```python
from build123d import *

# Parameters (mm, degrees)
SKETCH1_R            = 17.5
SKETCH1_R_2          = 15
BOSS_EXTRUDE1_DEPTH  = 80
CUT_SWEEP3_PROFILE_R = 2
FILLET2_R            = 2


with BuildPart() as part:
    # Sketch1 → Boss-Extrude1 (new body)
    with BuildSketch(Plane.XY):
        with BuildLine():
            Line((-17.5, 72.107864376), (-17.5, 63.75))
            Line((-17.5, 63.75), (-17.5, -66.25))
            Line((-17.5, -66.25), (-17.5, -76.567541634))
            ThreePointArc((-17.5, -76.567541634), (0, -106.25), (17.5, -76.567541634))
            Line((17.5, -76.567541634), (77.5, -76.567541634))
            Line((77.5, -76.567541634), (77.5, 72.107864376))
            Line((77.5, 72.107864376), (17.5, 72.107864376))
            ThreePointArc((17.5, 72.107864376), (0, 108.75), (-17.5, 72.107864376))
        make_face()
        with Locations((0, 86.25)):
            Circle(SKETCH1_R, mode=Mode.SUBTRACT)
        with Locations((0, -86.25)):
            Circle(SKETCH1_R_2, mode=Mode.SUBTRACT)
    extrude(amount=BOSS_EXTRUDE1_DEPTH)

    # Sketch9 → Cut-Revolve1 (revolve, cut)
    with BuildSketch(Plane.XY.offset(40), mode=Mode.PRIVATE) as cut_revolve1_sk:
        Polygon((-7.353554792, 47.770161371), (-7.353554792, 17.770161371), (6.646445208, 17.770161371), (6.646445208, 45.270161371), (12.283096941, 45.270161371), (12.283096941, 30.270161371), (62.283096941, 30.270161371), (62.283096941, 47.770161371), align=None)
    revolve(cut_revolve1_sk.sketch.rotate(Axis((-48.211470633, 47.770161371, 40), (1, 0, 0)), 270), axis=Axis((-48.211470633, 47.770161371, 40), (1, 0, 0)), mode=Mode.SUBTRACT)

    # Sketch38 → Cut-Revolve3 (revolve, cut)
    with BuildSketch(Plane.XY.offset(40), mode=Mode.PRIVATE) as cut_revolve3_sk:
        Polygon((17, 0), (17, 12.5), (22.475179435, 12.5), (22.475179435, 17.5), (102.052596933, 17.5), (102.052596933, 0), align=None)
    revolve(cut_revolve3_sk.sketch.rotate(Axis((102.052596933, 0, 40), (-1, 0, 0)), 90), axis=Axis((102.052596933, 0, 40), (-1, 0, 0)), mode=Mode.SUBTRACT)

    # Cut-Sweep3: sweep along a path in Sketch60
    with BuildLine(Plane.XY.offset(40)) as cut_sweep3_path:
        Line((57.751179251, 47.84482156), (68.211067836, 47.84482156))
        Line((68.211067836, 47.84482156), (68.211067836, 23.494918311))
        Line((68.211067836, 23.494918311), (19.159559926, 23.494918311))
        Line((19.159559926, 23.494918311), (19.159559926, 12.07117719))
    # Cut-Sweep3 profile (on start of the path) → Cut-Sweep3 (sweep, cut)
    with BuildSketch(Plane(origin=(57.751179251, 47.84482156, 40), x_dir=(0, 0, 1), z_dir=(1, 0, 0))):
        Circle(CUT_SWEEP3_PROFILE_R)
    sweep(path=cut_sweep3_path.line, transition=Transition.RIGHT, mode=Mode.SUBTRACT)

    # Fillet2
    fillet2_edges = [part.edges().sort_by_distance(p)[0] for p in [
        (47.5, -76.567541634, 0),
        (77.5, 72.107864376, 40),
        (77.5, -76.567541634, 40),
        (47.5, -76.567541634, 80),
        (77.5, -2.229838629, 80),
        (47.5, 72.107864376, 80),
        (47.5, 72.107864376, 0),
        (77.5, -2.229838629, 0),
    ]]
    fillet(fillet2_edges, radius=FILLET2_R)


solid = part.part
```
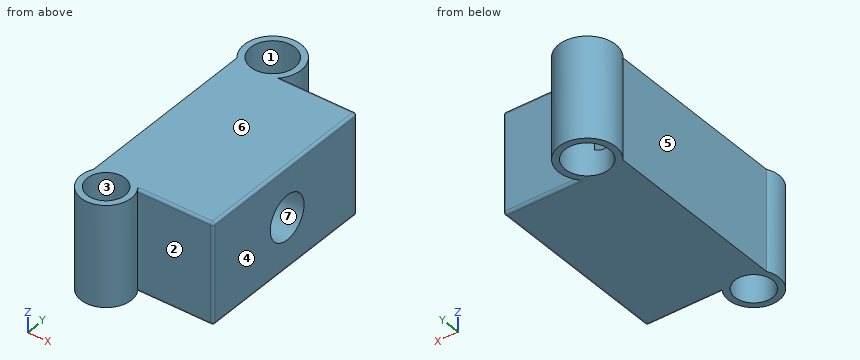
The listing builds one solid part. Answer for the finished solid, in the listing's coordinates (mm). Face numbers are marked on the shaded views. A direction names the side the tool comes from. Coordinates: 2 decimals unless noted, no trailing zeros. Write each loop counter-clockwise with the first axis right and the second up, starting at its lowest first coordinate (ties: lowest second). Pieces come first, ordered by that corner, then holes. Notation, with made-up numbers: M 80.25,23.5 L 126.25,23.5 A15 ccw 126.25,30.5 Z; hole C -34,-1 d8. An arc over 180 degrees is marked long. Use a Markdown table: item, result. Add a question column.
1. Straight lines are drawn through the part: line 1 along Y through (x, z) = (66, 40); line 2 along Y through (x, z) = (36, 40); line 3 along X through (y, z) = (41.5, 69). For each, find the intervals that lie inside material, in ascending order. Write a range as [from, to].
2. Section D-D (z = 17.5) is taken. Give the vertices of the cut face in (x, y).
3. Section B-B (x = 0) is taken. Give the vertices of the cut face in (y, z).
4. Section C-C (y = 37) is taken. Give the vertices of the cut face in (x, z), plus the area to 3 significant figures.
5. Given P1, Ø3, axis at x = -9, z = 13.5, coming from the +Y side; P2, Ø5, axis at y = 47.84, z = 40, coming from the -X side; P3, Ø10.5, axis at y = 8.5, z = 42, coming from the +X side, each flat-ended and moving along its own axis, determine where each tip first touches the part or whether it passes through.
6. For a pull along X with two mould halves and no side action, classify the marked faces 1, 2, 3 and 4 as +X half, -X half, draft (parallel to the pull), parting line (faces both ways), or undercut.
7. Which of the six approach directions +Z, -Z, +X, -X, +Y, -Y give full straight-line access (tool end or side, diameter ignored) to the marked faces 5, 6 and 7?
8. Section A-A (y = -86.25) is taken. Give the vertices of the cut face in (x, z).
Data:
| question | item | result |
|---|---|---|
| 1 | line 1 | y = [-76.57, -17.5], [17.5, 21.49], [25.49, 45.84], [49.84, 72.11] |
| 1 | line 2 | y = [-76.57, -17.5], [17.5, 21.49], [25.49, 30.27], [65.27, 72.11] |
| 1 | line 3 | x = [-17.5, -7.35], [6.65, 77.5] |
| 2 | outline | M -17.5,-76.57 A20 ccw long 17.5,-76.57 L 75.5,-76.57 A2 ccw 77.5,-74.57 L 77.5,70.11 A2 ccw 75.5,72.11 L 17.5,72.11 A22.5 ccw long -17.5,72.11 Z; hole C 0,86.25 d35; hole C 0,-86.25 d30; hole M -7.35,27.93 L 6.65,27.93 L 6.65,67.61 L -7.35,67.61 Z |
| 3 | outline | M -106.25,0 L -101.25,0 L -101.25,80 L -106.25,80 Z; M -71.25,0 L 68.75,0 L 68.75,18.56 A30 cw long 68.75,61.44 L 68.75,80 L -71.25,80 Z; M 103.75,0 L 108.75,0 L 108.75,80 L 103.75,80 Z |
| 4 | outline | M -17.5,0 L 75.5,0 A2 ccw 77.5,2 L 77.5,78 A2 ccw 75.5,80 L -17.5,80 Z; hole M -7.35,12 L 6.65,12 L 6.65,68 L -7.35,68 Z; hole M 12.28,26.21 L 62.28,26.21 L 62.28,53.79 L 12.28,53.79 Z; hole C 68.21,40 d4 |
| 4 | area | 5,420 mm2 |
| 5 | P1 | stops at y = 107.46 |
| 5 | P2 | stops at x = -17.5 |
| 5 | P3 | stops at x = 22.48 |
| 6 | face 1 | undercut |
| 6 | face 2 | draft |
| 6 | face 3 | undercut |
| 6 | face 4 | +X half |
| 7 | face 5 | +Z, -Z, -X |
| 7 | face 6 | +Z, +X, -X, +Y, -Y |
| 7 | face 7 | +X |
| 8 | outline | M -20,0 L -15,0 L -15,80 L -20,80 Z; M 15,0 L 20,0 L 20,80 L 15,80 Z |
